Build history of the part. All positions in model axes, mm. A direction names the side the tool comes from. Coordinates: 2 decimals unless noted, no trailing zeros. Order: outer loops, then holes, each group sorted by start corner. A loop starts at its lowest first (then second) coordinate and runs counter-clockwise, first axis right, second up. Notation, with made-up numbers: (-32.5, 40.5) - (-17.5, 40.5) arc R28 cw to (-17.5, 78.5) - close; hole circle Ø3 at (-11, -5). An arc over 180 degrees is marked (long way). Return JSON: item names as keys, results as strings.
Autodesk Inventor part; units mm, degrees
ref_plane "Work Plane1" through (0, 0, -27.5) normal (0, 0, -1) x (-1, 0, 0)
ref_plane "YZ Plane" through (0, 0, 0) normal (1, 0, 0) x (0, 1, 0)
ref_plane "XZ Plane" through (0, 0, 0) normal (0, 1, 0) x (-1, 0, 0)
sketch "Sketch1" plane through (0, 0, 0) normal (0, 1, 0) x (-1, 0, 0)
  line L0 (0, 0) -> (10, 0)
  line L1 (10, 0) -> (10, -55)
  line L2 (10, -55) -> (0, -55)
  line L3 (0, -55) -> (0, 0)
  line L4 (5, 0) -> (5, -6.5) construction
  line L5 (5, -6.5) -> (5, -48.5) construction
  circle A0 centre (5, -6.5) radius 2.25
  circle A1 centre (5, -48.5) radius 2.25
  line L6 (5, -27.5) -> (10, -27.5) construction
  line L7 (8.55, -4.4504) -> (8.55, -8.5496)
  line L8 (8.55, -8.5496) -> (5, -10.5992)
  line L9 (5, -10.5992) -> (1.45, -8.5496)
  line L10 (1.45, -8.5496) -> (1.45, -4.4504)
  line L11 (1.45, -4.4504) -> (5, -2.4008)
  line L12 (5, -2.4008) -> (8.55, -4.4504)
  line L13 (5, -44.4008) -> (8.55, -46.4504)
  line L14 (8.55, -46.4504) -> (8.55, -50.5496)
  line L15 (8.55, -50.5496) -> (5, -52.5992)
  line L16 (5, -52.5992) -> (1.45, -50.5496)
  line L17 (1.45, -50.5496) -> (1.45, -46.4504)
  line L18 (1.45, -46.4504) -> (5, -44.4008)
  line L19 (10, -27.5) -> (15, -27.5) construction
  line L20 (15, -27.5) -> (15, -17.5) construction
  line L21 (15, -27.5) -> (15, -37.5) construction
  circle A2 centre (15, -17.5) radius 2.25
  circle A3 centre (15, -37.5) radius 2.25
  line L22 (20, -17.5) -> (20, -37.5)
  line L23 (15, -27.5) -> (20, -27.5) construction
  line L24 (20, -17.5) -> (10, 0)
  line L25 (20, -37.5) -> (10, -55)
  circle A4 centre (15, -17.5) radius 4
  circle A5 centre (15, -37.5) radius 4
  line L26 (0, -27.5) -> (-5, -27.5) construction
  line L27 (-5, -27.5) -> (-5, -17.5) construction
  line L28 (-5, -27.5) -> (-5, -37.5) construction
  circle A6 centre (-5, -17.5) radius 2.25
  circle A7 centre (-5, -37.5) radius 2.25
  line L29 (-10, -17.5) -> (-10, -37.5)
  line L30 (-5, -27.5) -> (-10, -27.5) construction
  line L31 (-10, -17.5) -> (0, 0)
  line L32 (-10, -37.5) -> (0, -55)
  circle A8 centre (-5, -17.5) radius 4
  circle A9 centre (-5, -37.5) radius 4
  dimension "d2" = 10
  dimension "d3" = 55
  dimension "d4" = 7.1
  dimension "d5" = 7.1
  dimension "d6" = 42
  dimension "d7" = 4.5
  dimension "d12" = 20
  dimension "d13" = 4.5
  dimension "d15" = 20
  dimension "d16" = 8
  dimension "d17" = 8
  dimension "d18" = 10
extrude "Extrusion1" add sketch "Sketch1" along normal blind 4 contours L0 L1 L2 L3 | L7 L8 L9 L10 L11 L12 | L13 L14 L15 L16 L17 L18
extrude "Extrusion2" cut sketch "Sketch1" along normal blind 3 contours L7 L8 L9 L10 L11 L12 | L13 L14 L15 L16 L17 L18
ref_plane "Work Plane1" through (0, 0, -27.5) normal (0, 0, -1) x (-1, 0, 0)
sketch "Sketch2" plane through (0, 0, 0) normal (0, -1, 0) x (1, 0, 0)
  line L0 (-8.55, -4.4504) -> (-5, -2.4008)
  line L1 (-5, -2.4008) -> (-1.45, -4.4504)
  line L2 (-1.45, -4.4504) -> (-1.45, -8.5496)
  line L3 (-1.45, -8.5496) -> (-5, -10.5992)
  line L4 (-5, -10.5992) -> (-8.55, -8.5496)
  line L5 (-8.55, -8.5496) -> (-8.55, -4.4504)
  line L6 (-5, -44.4008) -> (-1.45, -46.4504)
  line L7 (-1.45, -46.4504) -> (-1.45, -50.5496)
  line L8 (-1.45, -50.5496) -> (-5, -52.5992)
  line L9 (-5, -52.5992) -> (-8.55, -50.5496)
  line L10 (-8.55, -50.5496) -> (-8.55, -46.4504)
  line L11 (-8.55, -46.4504) -> (-5, -44.4008)
  line L12 (0, -55) -> (-10, -55)
  line L13 (-10, 0) -> (0, 0)
  line L14 (4.2857, -7.5) -> (-14.2857, -7.5)
  line L15 (10, -27.5) -> (-20, -27.5) construction
  line L16 (0, 0) -> (0, -55)
  line L17 (-10, -55) -> (-10, 0)
  point P0 (-10, -7.5)
  point P1 (0, -7.5)
  dimension "d19" = 20
extrude "Extrusion3" add sketch "Sketch2" along normal blind 20 contours L5 L14 L17 L13 L16 L2 L1 L0 | L0 L1 L2 L14 L5
extrude "Extrusion4" cut sketch "Sketch1" against normal blind 4 contours A0 | L7 L8 L9 L10 L11 L12
chamfer "Chamfer1" distance 5 angle 45 1 edges at (-5, -4, -7.5)
sketch "Sketch3" plane through (-10, 4, 0) normal (0, 0, 1) x (1, 0, 0)
  line L0 (10, -24) -> (10, 0)
  line L1 (0, 0) -> (10, 0)
  line L2 (0, -24) -> (0, 0)
  line L3 (10, -24) -> (0, -24)
  line L4 (5, -24) -> (5, -14) construction
  circle A0 centre (5, -14) radius 2.25
  line L5 (10, -4) -> (0, -4)
  dimension "d27" = 10
  dimension "d28" = 4.5
extrude "Extrusion5" cut sketch "Sketch3" against normal through all contours A0
chamfer "Chamfer2" distance 5 angle 45 1 edges at (-5, -20, 0)
mirror "Mirror1" about plane through (0, 0, -27.5) normal (0, 0, -1) of "Extrusion5", "Extrusion3", "Extrusion4", "Chamfer1", "Chamfer2"
equation "\"d5\" = d4"
equation "\"d17\" = d16"
properties part number "Thread Bearing Bracket"
1. Cut at B-B on x = -6. State how many separate pieces and enclosed holes the cut face has, plus the area to 3 significant figures.
Check values:
{"separate pieces": "5", "enclosed holes": "0", "area": "324 mm²"}
2. Cut at C-C on y = -18. Give the cut face in (x, z), plus the area to 3 significant figures.
Check values:
{"outline": "(-10, -52) - (0, -52) - (0, -47.5) - (-10, -47.5) - close; (-10, -7.5) - (0, -7.5) - (0, -3) - (-10, -3) - close", "area": "90.0 mm²"}
3. Mould opens along Y. For faces 1 (the flat face through (-3.2, -0.54, -3.44)), 2 (the flat face through (-8.55, -2, -49)), 3 (the flat face through (-5, 4, -27)), 4 (the flat face through (-5, -6, 0)) say: pulls with the +Y half, pulls with the -Y half, needs draft (parallel to the pull), parting line crosses it, or undercut.
Check values:
{"face 1": "undercut", "face 2": "undercut", "face 3": "pulls with the +Y half", "face 4": "needs draft"}
4. Tool access for faces 5 (the flat face through (-5, -14, -7.5)), 6 (the flat face through (-3.2, 1.48, -45.44)), 7 (the flat face through (-6.8, -1.41, -51.56)), 8 (the cylindrical face through (-4.71, 3.49, -50.73)): list every direction of +Z, -Z, +X, -X, +Y, -Y with a clear straight run to the whole face (end or side of a thin tool).
Check values:
{"face 5": "+X, -X, -Y", "face 6": "-Y", "face 7": "none", "face 8": "+Y"}
5. Probe L1, parallel to Z at x = -5, y = 3.55; L2, parallel to Z at x = -3, y = 1; L3, parallel to Y at x = -6.5, z = -51.5. List the from-to ranges inside material, lowest first.
Check values:
{"L1": "-55 to -50.75, -46.25 to -8.75, -4.25 to 0", "L2": "-55 to -51.44, -45.56 to -9.44, -3.56 to 0", "L3": "-18.5 to -11.68, -8.32 to -5, 3 to 4"}
6. Drop a flat-ended pin along its axis: pin 1 (5 mm diameter, centred on x = -3, z = -28.5, fed in from -Y). Give the stop position or say it passes through.
Check values:
{"pin 1": "y = 0"}
7. Cut at A-A on y = -10. Give the cut face in (x, z).
Check values:
{"outline": "(-10, -55) - (-7.25, -55) - (-7.25, -47.5) - (-10, -47.5) - close; (-10, -7.5) - (-7.25, -7.5) - (-7.25, 0) - (-10, 0) - close; (-2.75, -55) - (0, -55) - (0, -47.5) - (-2.75, -47.5) - close; (-2.75, -7.5) - (0, -7.5) - (0, 0) - (-2.75, 0) - close"}
8. Cut at D-D on y = 1.5. Give the cut face in (x, z).
Check values:
{"outline": "(-10, -55) - (0, -55) - (0, 0) - (-10, 0) - close; hole (-8.55, -50.55) - (-5, -52.6) - (-1.45, -50.55) - (-1.45, -46.45) - (-5, -44.4) - (-8.55, -46.45) - close; hole (-8.55, -8.55) - (-5, -10.6) - (-1.45, -8.55) - (-1.45, -4.45) - (-5, -2.4) - (-8.55, -4.45) - close"}
